Design review of the part built by this model. Coordinates are the model's own, in mm. Give positions to 0.01 mm unless a question says otherwise; leave off trailing zeros. Loops run counter-clockwise (first coordinate to the right, second up) from the corner with the lowest first, then second, coordinate; pieces in that order, holes last. Notation, with made-up numbers: M 4.25,-1 L 25.25,-1 A19 ccw 25.25,8 Z; hole C 68,-4.75 d9. An arc over 180 degrees is marked long. Use one line per item in the form item = value. Start each with the question number.
from build123d import *

# Parameters (mm, degrees)
ESBO_O1_W                = 150
ESBO_O1_H                = 292
RESSALTO_EXTRUS_O1_DEPTH = 6
ESBO_O2_W                = 40
ESBO_O2_H                = 200
CORTE_EXTRUS_O1_DEPTH    = 329.329103188
ESBO_O5_W                = 20
ESBO_O5_H                = 6
ESBO_O5_W_2              = 85
CORTE_EXTRUS_O2_DEPTH    = 329.329103188
ESBO_O7_W                = 20
ESBO_O7_H                = 40
CORTE_EXTRUS_O3_DEPTH    = 329.329103188


with BuildPart() as part:
    # Esboço1 → Ressalto-extrusão1 (new body)
    with BuildSketch(Plane.XY):
        with Locations((75, 146)):
            Rectangle(ESBO_O1_W, ESBO_O1_H)
    extrude(amount=RESSALTO_EXTRUS_O1_DEPTH)

    # Esboço2 → Corte-extrusão1 (cut, through all)
    with BuildSketch(Plane(origin=(0, 0, 0), x_dir=(-1, 0, 0), z_dir=(0, 0, -1))):
        with Locations((-130, 147)):
            Rectangle(ESBO_O2_W, ESBO_O2_H)
    extrude(amount=-CORTE_EXTRUS_O1_DEPTH, mode=Mode.SUBTRACT)

    # Esboço5 → Corte-extrusão2 (cut, through all)
    with BuildSketch(Plane(origin=(0, 0, 0), x_dir=(-1, 0, 0), z_dir=(0, 0, -1))):
        with Locations((-125, 289)):
            Rectangle(ESBO_O5_W, ESBO_O5_H)
        with Locations((-57.5, 289)):
            Rectangle(ESBO_O5_W_2, ESBO_O5_H)
        with Locations((-125, 3)):
            Rectangle(ESBO_O5_W, ESBO_O5_H)
        with Locations((-57.5, 3)):
            Rectangle(ESBO_O5_W_2, ESBO_O5_H)
    extrude(amount=-CORTE_EXTRUS_O2_DEPTH, mode=Mode.SUBTRACT)

    # Esboço7 → Corte-extrusão3 (cut, through all)
    with BuildSketch(Plane(origin=(0, 0, 0), x_dir=(-1, 0, 0), z_dir=(0, 0, -1))):
        with Locations((-10, 227)):
            Rectangle(ESBO_O7_W, ESBO_O7_H)
    extrude(amount=-CORTE_EXTRUS_O3_DEPTH, mode=Mode.SUBTRACT)


solid = part.part
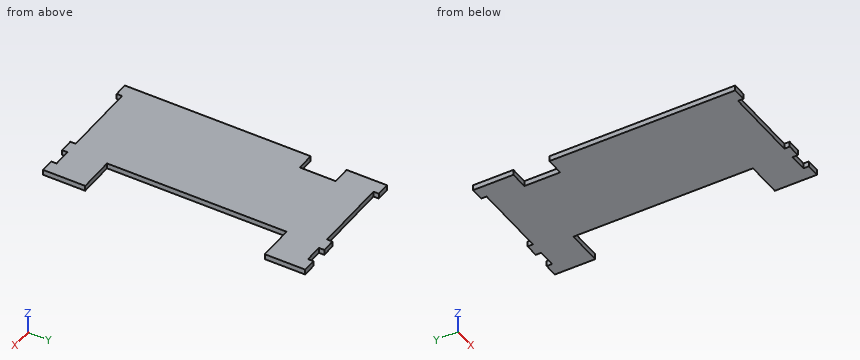
Q1. Clearance check with flat-ended pins moving along their axes: pin 1 Ø3 at (y, z) = (2, 2.5) entering from -X; pin 2 Ø2 at (y, z) = (213.5, 1.5) entering from +X; pin 3 Ø1.8 at (x, z) = (128.5, 4) entering from +Y; pin 4 Ø1.8 at (y, z) = (226, 4) entering from -X. State where each tip first meets the part, or that it passes through.
Q2. Take a section at A-A on z = 0.95. Give the boundary of the cut face in (x, y).
Q3. Take a section at B-B on y = 225. Give the boundary of the cut face in (x, z), plus the area to 3 significant figures.
Q4. Take a section at C-C on x = 55.5. Give the boundary of the cut face in (y, z), plus the area to 3 significant figures.
Q5. Wall thickness on probe 1 along Y at (x, z) = (9, 1.2); probe 2 along Y at (x, z) = (120, 2.45); probe 3 along Y at (x, z) = (63.5, 4.25): over which ranges is each line inside the solid? List them lowest first.
Response values:
q1.pin_1 = 0
q1.pin_2 = 110
q1.pin_3 = 286
q1.pin_4 = 20
q2.outline = M 0,0 L 15,0 L 15,6 L 100,6 L 100,0 L 115,0 L 115,6 L 135,6 L 135,0 L 150,0 L 150,47 L 110,47 L 110,247 L 150,247 L 150,292 L 135,292 L 135,286 L 115,286 L 115,292 L 100,292 L 100,286 L 15,286 L 15,292 L 0,292 L 0,247 L 20,247 L 20,207 L 0,207 Z
q3.outline = M 20,0 L 110,0 L 110,6 L 20,6 Z
q3.area = 540 mm^2
q4.outline = M 6,0 L 286,0 L 286,6 L 6,6 Z
q4.area = 1,680 mm^2
q5.probe_1 = 0 to 207, 247 to 292
q5.probe_2 = 6 to 47, 247 to 286
q5.probe_3 = 6 to 286
